Autodesk Inventor part; units mm, degrees
ref_plane "1NPN_XY" through (23, 22, -60) normal (0, 1, 0) x (1, 0, 0)
ref_plane "1NPN_YZ" through (23, 22, -60) normal (1, 0, 0) x (0, 0, -1)
ref_plane "1NPN_ZX" through (23, 22, -60) normal (0, 0, -1) x (0, 1, 0)
sketch "Sketch_1" plane through (0, 0, 0) normal (0, 0, 1) x (1, 0, 0)
  line L0 (0, 12) -> (0.2, 12)
  line L1 (0.2, 12) -> (0.2, 0)
  line L2 (0.2, 0) -> (3.5, 0)
  line L3 (3.5, 0) -> (3.5, 11.6)
  line L4 (3.5, 11.6) -> (42.5, 11.6)
  line L5 (42.5, 11.6) -> (42.5, 0)
  line L6 (42.5, 0) -> (72.6, 0)
  line L7 (72.6, 0) -> (72.6, 16.8029)
  arc A0 (72.6, 16.8029) -> (55, 21) centre (55, -18) ccw
  line L8 (55, 21) -> (46, 21)
  line L9 (46, 21) -> (46, 22)
  line L10 (46, 22) -> (0, 22)
  line L11 (0, 22) -> (0, 12)
extrude "Extrusion1" add sketch "Sketch_1" against normal blind 120
sketch "Sketch_2" plane through (0, 0, 0) normal (0, 0, 1) x (1, 0, 0)
  line L0 (-5, 27) -> (-5, -5)
  line L1 (-5, -5) -> (85, -5)
  line L2 (85, -5) -> (85, 27)
  line L3 (85, 27) -> (-5, 27)
  line L4 (0, 12) -> (0.2, 12)
  line L5 (0.2, 12) -> (0.2, 1)
  arc A0 (0.2, 1) -> (1.2, 0) centre (1.2, 1) ccw
  line L6 (1.2, 0) -> (72.6, 0)
  line L7 (72.6, 0) -> (72.6, 16.057)
  arc A1 (72.6, 16.057) -> (71.9206, 17.1382) centre (71.4, 16.057) ccw
  arc A2 (71.9206, 17.1382) -> (55, 21) centre (55, -18) ccw
  line L8 (55, 21) -> (46, 21)
  line L9 (46, 21) -> (46, 21.2)
  line L10 (46, 21.2) -> (45.2, 22)
  line L11 (45.2, 22) -> (1, 22)
  line L12 (1, 22) -> (0, 21)
  line L13 (0, 21) -> (0, 12)
extrude "Extrusion2" cut sketch "Sketch_2" against normal blind 120
sketch "Sketch_28" plane through (0, 0, -60) normal (0, 0, 1) x (1, 0, 0)
  line L0 (3.5, 11.6) -> (3.5, 0)
  line L1 (3.5, 0) -> (11, 0)
  line L2 (11, 0) -> (11, 5.5)
  line L3 (11, 5.5) -> (35, 5.5)
  line L4 (35, 5.5) -> (35, 0)
  line L5 (35, 0) -> (42.5, 0)
  line L6 (42.5, 0) -> (42.5, 11.6)
  line L7 (42.5, 11.6) -> (3.5, 11.6)
extrude "Extrusion3" add sketch "Sketch_28" along normal mid plane 120
sketch "Sketch_3" plane through (0, 0, -60) normal (0, 0, 1) x (1, 0, 0)
  line L0 (3.5, 11.6) -> (3.5, 0)
  line L1 (3.5, 0) -> (12.1883, 0)
  line L2 (12.1883, 0) -> (11.5169, 2.5055)
  arc A0 (11.5169, 2.5055) -> (11, 4.164) centre (10.73, 3.17) ccw
  line L3 (11, 4.164) -> (11, 4.9)
  line L4 (11, 4.9) -> (13.5186, 4.9)
  arc A1 (13.5186, 4.9) -> (15.064, 5.5) centre (14.07, 5.77) ccw
  line L5 (15.064, 5.5) -> (30.936, 5.5)
  arc A2 (30.936, 5.5) -> (32.4814, 4.9) centre (31.93, 5.77) ccw
  line L6 (32.4814, 4.9) -> (35, 4.9)
  line L7 (35, 4.9) -> (35, 4.164)
  arc A3 (35, 4.164) -> (34.4831, 2.5055) centre (35.27, 3.17) ccw
  line L8 (34.4831, 2.5055) -> (33.8117, 0)
  line L9 (33.8117, 0) -> (42.5, 0)
  line L10 (42.5, 0) -> (42.5, 11.6)
  line L11 (42.5, 11.6) -> (3.5, 11.6)
extrude "Extrusion4" add sketch "Sketch_3" along normal mid plane 120
sketch "Sketch_20" plane through (0, 0, 0) normal (0, 0, 1) x (1, 0, 0)
  line L0 (45.5, 3) -> (47.875, 3)
  line L1 (47.875, 3) -> (47.875, 0)
  line L2 (47.875, 0) -> (62.125, 0)
  line L3 (62.125, 0) -> (62.125, 3)
  line L4 (62.125, 3) -> (64.5, 3)
  line L5 (64.5, 3) -> (64.5, 9)
  line L6 (64.5, 9) -> (45.5, 9)
  line L7 (45.5, 9) -> (45.5, 3)
extrude "Extrusion5" cut sketch "Sketch_20" against normal blind 0.1
sketch "Sketch_21" plane through (0, 0, -120) normal (0, 0, 1) x (1, 0, 0)
  line L0 (45.5, 3) -> (47.875, 3)
  line L1 (47.875, 3) -> (47.875, 0)
  line L2 (47.875, 0) -> (62.125, 0)
  line L3 (62.125, 0) -> (62.125, 3)
  line L4 (62.125, 3) -> (64.5, 3)
  line L5 (64.5, 3) -> (64.5, 9)
  line L6 (64.5, 9) -> (45.5, 9)
  line L7 (45.5, 9) -> (45.5, 3)
extrude "Extrusion6" cut sketch "Sketch_21" along normal blind 0.1
sketch "Sketch7" plane through (72.6, 0, 0) normal (1, 0, 0) x (0, 0, -1)
  point P0 (21, 6)
hole "Hole1" at (72.6, 6, -21) direction (-1, 0, 0) diameter 3.242 depth 10 tip angle 120 countersink diameter 4 countersink angle 90
sketch "Sketch8" plane through (72.6, 0, 0) normal (1, 0, 0) x (0, 0, -1)
  point P0 (99, 6)
hole "Hole2" at (72.6, 6, -99) direction (-1, 0, 0) diameter 3.242 depth 10 tip angle 120 countersink diameter 4 countersink angle 90
sketch "Sketch_8" plane through (7, 0, 0) normal (1, 0, 0) x (0, 0, -1)
  line L0 (23, 14.5) -> (23, 22)
  line L1 (23, 22) -> (25.5, 22)
  line L2 (25.5, 22) -> (25.067, 21.567)
  line L3 (25.067, 21.567) -> (25.067, 14.5)
  line L4 (25.067, 14.5) -> (23, 14.5)
  line L5 (23, 14.5) -> (23, 22)
revolve "Revolution1" cut sketch "Sketch_8" angle 360 about axis through (7, 14.5, -23) along (0, -1, 0)
thread "Thread1"
sketch "Pattern_1_Sketch_8_0" plane through (39, 0, 0) normal (1, 0, 0) x (0, 0, -1)
  line L0 (23, 14.5) -> (23, 22)
  line L1 (23, 22) -> (25.5, 22)
  line L2 (25.5, 22) -> (25.067, 21.567)
  line L3 (25.067, 21.567) -> (25.067, 14.5)
  line L4 (25.067, 14.5) -> (23, 14.5)
  line L5 (23, 14.5) -> (23, 22)
revolve "Revolution2" cut sketch "Pattern_1_Sketch_8_0" angle 360 about axis through (39, 14.5, -23) along (0, -1, 0)
thread "Thread2"
sketch "Pattern_1_Sketch_8_1" plane through (39, 0, 0) normal (1, 0, 0) x (0, 0, -1)
  line L0 (38, 14.5) -> (38, 22)
  line L1 (38, 22) -> (40.5, 22)
  line L2 (40.5, 22) -> (40.067, 21.567)
  line L3 (40.067, 21.567) -> (40.067, 14.5)
  line L4 (40.067, 14.5) -> (38, 14.5)
  line L5 (38, 14.5) -> (38, 22)
revolve "Revolution3" cut sketch "Pattern_1_Sketch_8_1" angle 360 about axis through (39, 14.5, -38) along (0, -1, 0)
thread "Thread3"
sketch "Pattern_1_Sketch_8_2" plane through (7, 0, 0) normal (1, 0, 0) x (0, 0, -1)
  line L0 (38, 14.5) -> (38, 22)
  line L1 (38, 22) -> (40.5, 22)
  line L2 (40.5, 22) -> (40.067, 21.567)
  line L3 (40.067, 21.567) -> (40.067, 14.5)
  line L4 (40.067, 14.5) -> (38, 14.5)
  line L5 (38, 14.5) -> (38, 22)
revolve "Revolution4" cut sketch "Pattern_1_Sketch_8_2" angle 360 about axis through (7, 14.5, -38) along (0, -1, 0)
thread "Thread4"
sketch "Pattern_1_Sketch_8_3" plane through (39, 0, 0) normal (1, 0, 0) x (0, 0, -1)
  line L0 (82, 14.5) -> (82, 22)
  line L1 (82, 22) -> (84.5, 22)
  line L2 (84.5, 22) -> (84.067, 21.567)
  line L3 (84.067, 21.567) -> (84.067, 14.5)
  line L4 (84.067, 14.5) -> (82, 14.5)
  line L5 (82, 14.5) -> (82, 22)
revolve "Revolution5" cut sketch "Pattern_1_Sketch_8_3" angle 360 about axis through (39, 14.5, -82) along (0, -1, 0)
thread "Thread5"
sketch "Pattern_1_Sketch_8_4" plane through (7, 0, 0) normal (1, 0, 0) x (0, 0, -1)
  line L0 (82, 14.5) -> (82, 22)
  line L1 (82, 22) -> (84.5, 22)
  line L2 (84.5, 22) -> (84.067, 21.567)
  line L3 (84.067, 21.567) -> (84.067, 14.5)
  line L4 (84.067, 14.5) -> (82, 14.5)
  line L5 (82, 14.5) -> (82, 22)
revolve "Revolution6" cut sketch "Pattern_1_Sketch_8_4" angle 360 about axis through (7, 14.5, -82) along (0, -1, 0)
thread "Thread6"
sketch "Pattern_1_Sketch_8_5" plane through (39, 0, 0) normal (1, 0, 0) x (0, 0, -1)
  line L0 (97, 14.5) -> (97, 22)
  line L1 (97, 22) -> (99.5, 22)
  line L2 (99.5, 22) -> (99.067, 21.567)
  line L3 (99.067, 21.567) -> (99.067, 14.5)
  line L4 (99.067, 14.5) -> (97, 14.5)
  line L5 (97, 14.5) -> (97, 22)
revolve "Revolution7" cut sketch "Pattern_1_Sketch_8_5" angle 360 about axis through (39, 14.5, -97) along (0, -1, 0)
thread "Thread7"
sketch "Pattern_1_Sketch_8_6" plane through (7, 0, 0) normal (1, 0, 0) x (0, 0, -1)
  line L0 (97, 14.5) -> (97, 22)
  line L1 (97, 22) -> (99.5, 22)
  line L2 (99.5, 22) -> (99.067, 21.567)
  line L3 (99.067, 21.567) -> (99.067, 14.5)
  line L4 (99.067, 14.5) -> (97, 14.5)
  line L5 (97, 14.5) -> (97, 22)
revolve "Revolution8" cut sketch "Pattern_1_Sketch_8_6" angle 360 about axis through (7, 14.5, -97) along (0, -1, 0)
thread "Thread8"
sketch "Sketch_10" plane through (23, 0, 0) normal (1, 0, 0) x (0, 0, -1)
  line L0 (40, 19.9) -> (40, 13.4)
  line L1 (40, 13.4) -> (37.5415, 13.4)
  line L2 (37.5415, 13.4) -> (37.5415, 19.3585)
  line L3 (37.5415, 19.3585) -> (37, 19.9)
  line L4 (37, 19.9) -> (35.5, 19.9)
  line L5 (35.5, 19.9) -> (35.5, 22)
  line L6 (35.5, 22) -> (40, 22)
  line L7 (40, 22) -> (40, 13.4)
revolve "Revolution9" cut sketch "Sketch_10" angle 360 about axis through (23, 19.9, -40) along (0, 1, 0)
thread "Thread9"
sketch "Sketch_11" plane through (23, 0, 0) normal (1, 0, 0) x (0, 0, -1)
  line L0 (80, 19.9) -> (80, 13.4)
  line L1 (80, 13.4) -> (77.5415, 13.4)
  line L2 (77.5415, 13.4) -> (77.5415, 19.3585)
  line L3 (77.5415, 19.3585) -> (77, 19.9)
  line L4 (77, 19.9) -> (75.5, 19.9)
  line L5 (75.5, 19.9) -> (75.5, 22)
  line L6 (75.5, 22) -> (80, 22)
  line L7 (80, 22) -> (80, 13.4)
revolve "Revolution10" cut sketch "Sketch_11" angle 360 about axis through (23, 19.9, -80) along (0, 1, 0)
thread "Thread10"
sketch "Sketch27" plane through (0, 12, -120) normal (-1, 0, 0) x (0, 0, 1)
  point P0 (75, 5)
hole "Hole3" at (0, 17, -45) direction (1, 0, 0) diameter 4.134 depth 14 tip angle 120 countersink diameter 5 countersink angle 90
sketch "Sketch28" plane through (0, 12, -120) normal (-1, 0, 0) x (0, 0, 1)
  point P0 (45, 5)
hole "Hole4" at (0, 17, -75) direction (1, 0, 0) diameter 4.134 depth 14 tip angle 120 countersink diameter 5 countersink angle 90
sketch "Sketch_14" plane through (0, 17, 0) normal (0, 1, 0) x (1, 0, 0)
  line L0 (2.1, 30) -> (0, 30)
  line L1 (0, 30) -> (0, 33.5)
  line L2 (0, 33.5) -> (2.1, 33.5)
  line L3 (2.1, 33.5) -> (2.1, 30)
  line L4 (2.1, 30) -> (0, 30)
revolve "Revolution11" cut sketch "Sketch_14" angle 360 about axis through (2.1, 17, -30) along (1, 0, 0)
sketch "Sketch_15" plane through (0, 17, 0) normal (0, 1, 0) x (1, 0, 0)
  line L0 (2.1, 90) -> (0, 90)
  line L1 (0, 90) -> (0, 93.5)
  line L2 (0, 93.5) -> (2.1, 93.5)
  line L3 (2.1, 93.5) -> (2.1, 90)
  line L4 (2.1, 90) -> (0, 90)
revolve "Revolution12" cut sketch "Sketch_15" angle 360 about axis through (2.1, 17, -90) along (1, 0, 0)
ref_plane "1NPN_XY" through (23, 22, -60) normal (0, 1, 0) x (1, 0, 0)
ref_plane "1NPN_YZ" through (23, 22, -60) normal (1, 0, 0) x (0, 0, -1)
ref_plane "1NPN_ZX" through (23, 22, -60) normal (0, 0, -1) x (0, 1, 0)
ref_plane "BP1_1_XY" through (3.5, 13.5, 6.5) normal (1, 0, 0) x (0, 0, -1)
ref_plane "BP1_1_YZ" through (3.5, 13.5, 6.5) normal (0, 0, -1) x (0, 1, 0)
ref_plane "BP1_1_ZX" through (3.5, 13.5, 6.5) normal (0, 1, 0) x (1, 0, 0)
ref_plane "BP1_2_XY" through (3.5, 13.5, -126.5) normal (1, 0, 0) x (0, 0, -1)
ref_plane "BP1_2_YZ" through (3.5, 13.5, -126.5) normal (0, 0, -1) x (0, 1, 0)
ref_plane "BP1_2_ZX" through (3.5, 13.5, -126.5) normal (0, 1, 0) x (1, 0, 0)
ref_plane "BP2_1_XY" through (42.5, 13.5, 6.5) normal (1, 0, 0) x (0, 0, -1)
ref_plane "BP2_1_YZ" through (42.5, 13.5, 6.5) normal (0, 0, -1) x (0, 1, 0)
ref_plane "BP2_1_ZX" through (42.5, 13.5, 6.5) normal (0, 1, 0) x (1, 0, 0)
ref_plane "BP2_2_XY" through (42.5, 13.5, -126.5) normal (1, 0, 0) x (0, 0, -1)
ref_plane "BP2_2_YZ" through (42.5, 13.5, -126.5) normal (0, 0, -1) x (0, 1, 0)
ref_plane "BP2_2_ZX" through (42.5, 13.5, -126.5) normal (0, 1, 0) x (1, 0, 0)
ref_plane "BP3_XY" through (23, 21, 6.5) normal (0, 1, 0) x (1, 0, 0)
ref_plane "BP3_YZ" through (23, 21, 6.5) normal (1, 0, 0) x (0, 0, -1)
ref_plane "BP3_ZX" through (23, 21, 6.5) normal (0, 0, -1) x (0, 1, 0)
ref_plane "BP5_XY" through (23, 21, -126.5) normal (0, 1, 0) x (1, 0, 0)
ref_plane "BP5_YZ" through (23, 21, -126.5) normal (1, 0, 0) x (0, 0, -1)
ref_plane "BP5_ZX" through (23, 21, -126.5) normal (0, 0, -1) x (0, 1, 0)
ref_plane "EXPT_BLOCK_XY" through (23, 22, -40) normal (0, -1, 0) x (1, 0, 0)
ref_plane "EXPT_BLOCK_YZ" through (23, 22, -40) normal (1, 0, 0) x (0, 0, 1)
ref_plane "EXPT_BLOCK_ZX" through (23, 22, -40) normal (0, 0, 1) x (0, -1, 0)
ref_plane "EXPT_HALTEWINKEL_H_XY" through (0, 17, -60) normal (1, 0, 0) x (0, 0, -1)
ref_plane "EXPT_HALTEWINKEL_H_YZ" through (0, 17, -60) normal (0, 0, -1) x (0, 1, 0)
ref_plane "EXPT_HALTEWINKEL_H_ZX" through (0, 17, -60) normal (0, 1, 0) x (1, 0, 0)
ref_plane "EXPT_HALTEWINKEL_V_XY" through (72.6, 6, -60) normal (-1, 0, 0) x (0, 0, -1)
ref_plane "EXPT_HALTEWINKEL_V_YZ" through (72.6, 6, -60) normal (0, 0, -1) x (0, -1, 0)
ref_plane "EXPT_HALTEWINKEL_V_ZX" through (72.6, 6, -60) normal (0, -1, 0) x (-1, 0, 0)
ref_plane "SCHALTFAHNE_XY" through (72.6, 6, -60) normal (-1, 0, 0) x (0, 0, -1)
ref_plane "SCHALTFAHNE_YZ" through (72.6, 6, -60) normal (0, 0, -1) x (0, -1, 0)
ref_plane "SCHALTFAHNE_ZX" through (72.6, 6, -60) normal (0, -1, 0) x (-1, 0, 0)
ref_plane "SCHLITTEN_XY" through (23, -1.5, -60) normal (0, 0, -1) x (1, 0, 0)
ref_plane "SCHLITTEN_YZ" through (23, -1.5, -60) normal (1, 0, 0) x (0, -1, 0)
ref_plane "SCHLITTEN_ZX" through (23, -1.5, -60) normal (0, -1, 0) x (0, 0, -1)
ref_plane "SENSOR_XY" through (0, 17, -75) normal (1, 0, 0) x (0, 0, -1)
ref_plane "SENSOR_YZ" through (0, 17, -75) normal (0, 0, -1) x (0, 1, 0)
ref_plane "SENSOR_ZX" through (0, 17, -75) normal (0, 1, 0) x (1, 0, 0)
properties part number "EGC-80-GK-GPTB1--------(0)"
Input: part model. Units: mm. Frame: model coordinates. A direction names the side the tool comes from. Round coordinates to 2 decimals unless told otherwise and drop trailing zeros. Order: outer loops, then holes, each group sorted by start corner. A loop starts at its lowest first (then second) coordinate and runs counter-clockwise, first axis right, second up.
1. Pin query (flat end, axial travel): P1, Ø2.5, axis at x = 39, z = -82, coming from the +Y side; P2, Ø10, axis at x = 18.5, z = -31.5, coming from the -Y side; P3, Ø5.5, axis at x = 23, z = -80, coming from the -Y side. Return the tip coordinate at first contact, or that it passes through.
The answers:
P1: stops at y = 14.5
P2: stops at y = 4.74
P3: stops at y = 5.5
2. Material intervals for line 1 (X direction, y = 16, z = -38); line 2 (X direction, y = 1.5, z = -32.5); line 3 (Y direction, x = 53.5, z = -104), sorted ascending.
The answers:
line 1: x = 0 to 4.93, 9.07 to 21.57, 24.43 to 36.93, 41.07 to 72.6
line 2: x = 0.2 to 11.79, 34.21 to 72.6
line 3: y = 0 to 21
3. Mould query, pull axis X, two halves, no side actions, for faces 1 (the face through (2.1, 17, -30)), 2 (the face through (7, 14.5, -23)), 3 (the face through (20, 19.9, -39)), 4 (the face through (1.06, 19.95, -31.88)). Classes: released by +X, released by -X, zero draft, split by the parting line, or undercut.
The answers:
face 1: released by -X
face 2: undercut
face 3: undercut
face 4: zero draft
4. Cut plane B-B, the plane z = -16. Output: boundary loops of the cut face in (x, y).
The answers:
outline: (0, 12) - (0.2, 12) - (0.2, 1) arc R1 ccw to (1.2, 0) - (12.19, 0) - (11.52, 2.51) arc R1.03 ccw to (11, 4.16) - (11, 4.9) - (13.52, 4.9) arc R1.03 ccw to (15.06, 5.5) - (30.94, 5.5) arc R1.03 ccw to (32.48, 4.9) - (35, 4.9) - (35, 4.16) arc R1.03 ccw to (34.48, 2.51) - (33.81, 0) - (72.6, 0) - (72.6, 16.06) arc R1.2 ccw to (71.92, 17.14) arc R39 ccw to (55, 21) - (46, 21) - (46, 21.2) - (45.2, 22) - (1, 22) - (0, 21) - close
5. Set-up query: faces 5 (the face through (23, 22, -59)), 6 (the face through (0.2, 7, -59)), 7 (the face through (39.091, 17.984, -94.935)), 8 (the face through (63.797, 19.995, -59.16)), 9 (the face through (67.343, 5.513, -100.546)). Return all of +Z, -Z, +X, -X, +Y, -Y with unobstructed straight access to the full face (end or side cutting, diameter ignored); none if empty.
The answers:
face 5: +Z, -Z, +X, -X, +Y
face 6: +Z, -Z, -X, -Y
face 7: +Y
face 8: +Z, -Z, +X, +Y
face 9: +X
6. Cut plane A-A, the plane x = 39. Output: boundary loops of the cut face in (y, z).
The answers:
outline: (0, -120) - (22, -120) - (22, -99.5) - (21.57, -99.07) - (14.5, -99.07) - (14.5, -94.93) - (21.57, -94.93) - (22, -94.5) - (22, -84.5) - (21.57, -84.07) - (14.5, -84.07) - (14.5, -79.93) - (21.57, -79.93) - (22, -79.5) - (22, -40.5) - (21.57, -40.07) - (14.5, -40.07) - (14.5, -35.93) - (21.57, -35.93) - (22, -35.5) - (22, -25.5) - (21.57, -25.07) - (14.5, -25.07) - (14.5, -20.93) - (21.57, -20.93) - (22, -20.5) - (22, 0) - (0, 0) - close
